from build123d import *

# Parameters (mm, degrees)
SKETCH1_R           = 295
SKETCH1_R_2         = 165
BOSS_EXTRUDE1_DEPTH = 6.7
SKETCH2_W           = 6.7
SKETCH2_H           = 34
SKETCH2_H_2         = 44
CUT_EXTRUDE3_DEPTH  = 6.7
SKETCH3_R           = 280
SKETCH3_R_2         = 273.8
SKETCH3_R_3         = 12
CUT_EXTRUDE4_DEPTH  = 2.5
SKETCH5_R           = 296
SKETCH5_R_2         = 285
CUT_EXTRUDE5_DEPTH  = 3.5


with BuildPart() as part:
    # Sketch1 → Boss-Extrude1 (new body)
    with BuildSketch(Plane(origin=(0, 0, 0), x_dir=(1, 0, 0), z_dir=(0, 1, 0))):
        with Locations(Location((0, 0, 0), (0, 0, 270))):
            Circle(SKETCH1_R)
        with Locations(Location((0, 0, 0), (0, 0, 270))):
            Circle(SKETCH1_R_2, mode=Mode.SUBTRACT)
    extrude(amount=BOSS_EXTRUDE1_DEPTH)

    # Sketch2 → Cut-Extrude3 (cut)
    with BuildSketch(Plane(origin=(0, 6.7, 0), x_dir=(1, 0, 0), z_dir=(0, 1, 0))):
        Polygon((254.66851952, 150.901185103), (216.563401754, 128.901185103), (219.913401754, 123.098814897), (258.01851952, 145.098814897), align=None)
        Polygon((169.798029949, 101.901185103), (140.353166221, 84.901185103), (143.703166221, 79.098814897), (173.148029949, 96.098814897), align=None)
        Polygon((129.838195602, -149.523461245), (107.983416873, -123.477950179), (102.850919104, -127.784627164), (124.705697833, -153.83013823), align=None)
        Polygon((290.921373496, -54.698966562), (292.084816287, -48.100754617), (248.753275154, -40.460234799), (247.589832364, -47.058446745), align=None)
        Polygon((195.573656492, -31.083233205), (162.090192889, -25.179195165), (160.926750099, -31.77740711), (194.410213701, -37.681445151), align=None)
        Polygon((187.698883583, -228.902493656), (192.831381352, -224.595816671), (164.548726525, -190.889861174), (159.416228757, -195.196538158), align=None)
        with Locations((0, -181)):
            Rectangle(SKETCH2_W, SKETCH2_H)
        with Locations((0, -274)):
            Rectangle(SKETCH2_W, SKETCH2_H_2)
        Polygon((-124.705697833, -153.83013823), (-102.850919104, -127.784627164), (-107.983416873, -123.477950179), (-129.838195602, -149.523461245), align=None)
        Polygon((-192.831381352, -224.595816671), (-187.698883583, -228.902493656), (-159.416228757, -195.196538158), (-164.548726525, -190.889861174), align=None)
        Polygon((-194.410213701, -37.681445151), (-160.926750099, -31.77740711), (-162.090192889, -25.179195165), (-195.573656492, -31.083233205), align=None)
        Polygon((-292.084816287, -48.100754617), (-290.921373496, -54.698966562), (-247.589832364, -47.058446745), (-248.753275154, -40.460234799), align=None)
        Polygon((-254.66851952, 150.901185103), (-258.01851952, 145.098814897), (-219.913401754, 123.098814897), (-216.563401754, 128.901185103), align=None)
        Polygon((-173.148029949, 96.098814897), (-143.703166221, 79.098814897), (-140.353166221, 84.901185103), (-169.798029949, 101.901185103), align=None)
    extrude(amount=-CUT_EXTRUDE3_DEPTH, mode=Mode.SUBTRACT)

    # Sketch3 → Cut-Extrude4 (cut)
    # profile 1 of 10: a face of its own
    with BuildSketch(Plane(origin=(0, 6.7, 0), x_dir=(1, 0, 0), z_dir=(0, 1, 0))):
        Circle(SKETCH3_R)
        Circle(SKETCH3_R_2, mode=Mode.SUBTRACT)
    # profile 2 of 10: a face of its own
    with BuildSketch(Plane(origin=(0, 6.7, 0), x_dir=(1, 0, 0), z_dir=(0, 1, 0))):
        with Locations(Location((0, -225, 0), (0, 0, 270))):
            Circle(SKETCH3_R_3)
    # profile 3 of 10: a face of its own
    with BuildSketch(Plane(origin=(0, 6.7, 0), x_dir=(1, 0, 0), z_dir=(0, 1, 0))):
        with Locations(Location((-144.627212179, -172.359999702, 0), (0, 0, 270))):
            Circle(SKETCH3_R_3)
    # profile 4 of 10: a face of its own
    with BuildSketch(Plane(origin=(0, 6.7, 0), x_dir=(1, 0, 0), z_dir=(0, 1, 0))):
        with Locations(Location((-221.581744428, -39.070839975, 0), (0, 0, 270))):
            Circle(SKETCH3_R_3)
    # profile 5 of 10: a face of its own
    with BuildSketch(Plane(origin=(0, 6.7, 0), x_dir=(1, 0, 0), z_dir=(0, 1, 0))):
        with Locations(Location((-194.855715851, 112.5, 0), (0, 0, 270))):
            Circle(SKETCH3_R_3)
    # profile 6 of 10: a face of its own
    with BuildSketch(Plane(origin=(0, 6.7, 0), x_dir=(1, 0, 0), z_dir=(0, 1, 0))):
        with Locations(Location((-76.954532248, 211.430839677, 0), (0, 0, 270))):
            Circle(SKETCH3_R_3)
    # profile 7 of 10: a face of its own
    with BuildSketch(Plane(origin=(0, 6.7, 0), x_dir=(1, 0, 0), z_dir=(0, 1, 0))):
        with Locations(Location((76.954532248, 211.430839677, 0), (0, 0, 270))):
            Circle(SKETCH3_R_3)
    # profile 8 of 10: a face of its own
    with BuildSketch(Plane(origin=(0, 6.7, 0), x_dir=(1, 0, 0), z_dir=(0, 1, 0))):
        with Locations(Location((194.855715851, 112.5, 0), (0, 0, 270))):
            Circle(SKETCH3_R_3)
    # profile 9 of 10: a face of its own
    with BuildSketch(Plane(origin=(0, 6.7, 0), x_dir=(1, 0, 0), z_dir=(0, 1, 0))):
        with Locations(Location((221.581744428, -39.070839975, 0), (0, 0, 270))):
            Circle(SKETCH3_R_3)
    # profile 10 of 10: a face of its own
    with BuildSketch(Plane(origin=(0, 6.7, 0), x_dir=(1, 0, 0), z_dir=(0, 1, 0))):
        with Locations(Location((144.627212179, -172.359999702, 0), (0, 0, 270))):
            Circle(SKETCH3_R_3)
    extrude(amount=-CUT_EXTRUDE4_DEPTH, mode=Mode.SUBTRACT)

    # Sketch5 → Cut-Extrude5 (cut)
    with BuildSketch(Plane(origin=(0, 6.7, 0), x_dir=(1, 0, 0), z_dir=(0, 1, 0))):
        Circle(SKETCH5_R)
        Circle(SKETCH5_R_2, mode=Mode.SUBTRACT)
    extrude(amount=-CUT_EXTRUDE5_DEPTH, mode=Mode.SUBTRACT)


solid = part.part
Can you work these out from the model? Positions are in its coordinate system, mm. A direction names the side the tool comes from. Coordinates: 2 decimals unless noted, no trailing zeros. Loops run counter-clockwise (first coordinate to the right, second up) from the corner with the lowest first, then second, coordinate; pieces in that order, holes last. Notation, with made-up numbers: M 25,-24 L 58,-24 A21 ccw 58,-2 Z; hole C 22.5,82.25 d2. An arc over 180 degrees is marked long. Return JSON: item names as keys, results as strings. Group by question number.
Item 1: I'm going to push flat-ended pins straight in: pin 1 Ø4 at (y, z) = (6, -5) entering from -X; pin 2 Ø21.5 at (x, z) = (76.95, -211.43) entering from +Y. Where does each tip first touch, or does it pass through?
Item 2: If I drill on L1, parallel to X at y = 4.85, z = -112.5; L2, parallel to X at y = 5.5, z = -132; L3, parallel to Z at x = 180, y = 5.5, over which ranges is the centre line in solid material (lowest first)? Write a range as from..to.
Item 3: Thinking about a two-plate mould opening in X: for faces 1 (the flat face through (95, 3.2, 271)), 2 (the cylindrical face through (246.142, 4.974, 143.664)), 3 (the cylindrical face through (92.431, 5.468, 257.727)), 4 (the flat face through (-230.78, 3.4, -137.11)), which applies, released by +X, released by -X, zero draft, split by the parting line, or undercut?
Item 4: Imagine slicing it at C-C (z = 16). Please give me the cut outline in (x, y), and give its area (3 significant figures).
Item 5: Imagine slicing it at A-A (z = 172.36). Please give me the cut outline in (x, y), and give its area (3 significant figures).
Item 6: Imagine slicing it at D-D (z = -112.5). Please give me the cut outline in (x, y).
Item 7: On a 3-axis mill with a long thin cutter (end or side, diameter ignored), from which of +Z, -Z, +X, -X, +Y, -Y can I reach the whole of each face in a straight line? I mean faces 5 (the flat face through (155.694, 3.397, -93.758)), 6 (the cylindrical face through (4.13, 4.97, -284.97)), 7 (the cylindrical face through (-94.857, 5.468, 256.843)). Say none if no direction works.
Item 8: Imagine slicing it at B-B (z = -180.5). Please give me the cut outline in (x, y).
Verdict:
{
 "1": {"pin 1": "stops at x = -284.98", "pin 2": "stops at y = 4.2"},
 "2": {"L1": "x = -261.86..-256.41, -249.62..-206.86, -182.86..-120.7, 120.7..182.86, 206.86..249.62, 256.41..261.86", "L2": "x = -252.59..-246.93, -239.88..-235.33, -221.93..-99, 99..221.93, 235.33..239.88, 246.93..252.59", "L3": "z = -220.96..-214.48, -206.32..28.34, 35.14..206.32, 219.73..220.96"},
 "3": {"face 1": "zero draft", "face 2": "released by +X", "face 3": "undercut", "face 4": "undercut"},
 "4": {"outline": "M -294.57,0 L -164.22,0 L -164.22,6.7 L -273.33,6.7 L -273.33,4.2 L -279.54,4.2 L -279.54,6.7 L -284.55,6.7 L -284.55,3.2 L -294.57,3.2 Z; M 164.22,0 L 294.57,0 L 294.57,3.2 L 284.55,3.2 L 284.55,6.7 L 279.54,6.7 L 279.54,4.2 L 273.33,4.2 L 273.33,6.7 L 164.22,6.7 Z", "area": "1,650 mm^2"},
 "5": {"outline": "M -239.41,0 L -3.35,0 L -3.35,6.7 L -132.63,6.7 L -132.63,4.2 L -156.63,4.2 L -156.63,6.7 L -212.74,6.7 L -212.74,4.2 L -220.66,4.2 L -220.66,6.7 L -226.97,6.7 L -226.97,3.2 L -239.41,3.2 Z; M 3.35,0 L 239.41,0 L 239.41,3.2 L 226.97,3.2 L 226.97,6.7 L 220.66,6.7 L 220.66,4.2 L 212.74,4.2 L 212.74,6.7 L 156.63,6.7 L 156.63,4.2 L 132.63,4.2 L 132.63,6.7 L 3.35,6.7 Z", "area": "2,920 mm^2"},
 "6": {"outline": "M -272.71,0 L -120.7,0 L -120.7,6.7 L -182.86,6.7 L -182.86,4.2 L -206.86,4.2 L -206.86,6.7 L -249.62,6.7 L -249.62,4.2 L -256.41,4.2 L -256.41,6.7 L -261.86,6.7 L -261.86,3.2 L -272.71,3.2 Z; M 120.7,0 L 272.71,0 L 272.71,3.2 L 261.86,3.2 L 261.86,6.7 L 256.41,6.7 L 256.41,4.2 L 249.62,4.2 L 249.62,6.7 L 206.86,6.7 L 206.86,4.2 L 182.86,4.2 L 182.86,6.7 L 120.7,6.7 Z"},
 "7": {"face 5": "+Y, -Y", "face 6": "-Z, +Y", "face 7": "+Y"},
 "8": {"outline": "M -233.33,0 L 233.33,0 L 233.33,3.2 L 220.56,3.2 L 220.56,6.7 L 214.06,6.7 L 214.06,4.2 L 205.88,4.2 L 205.88,6.7 L -205.88,6.7 L -205.88,4.2 L -214.06,4.2 L -214.06,6.7 L -220.56,6.7 L -220.56,3.2 L -233.33,3.2 Z"}
}
